Part model, mm, in its own coordinate system. Face numbers are marked on the shaded views. A direction names the side the tool comes from. Coordinates: 2 decimals unless noted, no trailing zeros. Loops run counter-clockwise (first coordinate to the right, second up) from the corner with the lowest first, then second, coordinate; pieces in that order, holes last. Notation, with made-up numbers: M 2.5,33 L 20.5,33 A17 cw 20.5,39 Z; hole C 23.25,-13.5 d2. An arc over 180 degrees is marked long. Answer as CSV lines item,"result". Start each with the question number.
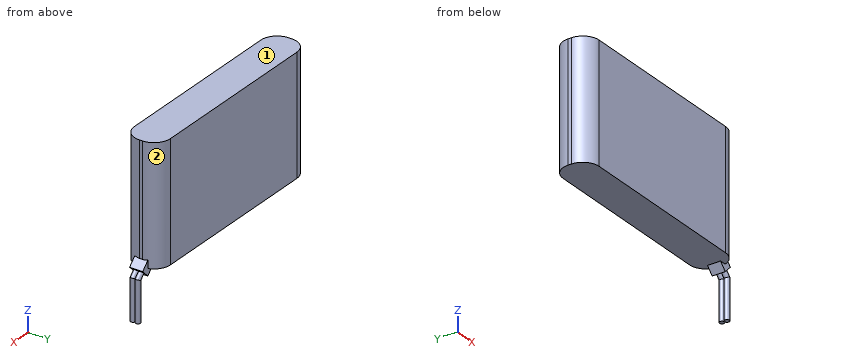
from build123d import *

# Parameters (mm, degrees)
SKETCH_1_W         = 130
SKETCH_1_H         = 72
EXTRUDE_1_DEPTH    = 22
FILLET_2_R         = 10
EXTRUDE_2_DEPTH    = 4
SWEEP_15_PROFILE_R = 1.475


with BuildPart() as part:
    # 草图1 → 凸台-拉伸1 (new body)
    with BuildSketch(Plane(origin=(0, 0, 0), x_dir=(1, 0, 0), z_dir=(0, 1, 0))):
        with Locations((2.770491803, 5.131147541)):
            Rectangle(SKETCH_1_W, SKETCH_1_H)
    extrude(amount=EXTRUDE_1_DEPTH)

    # 圆角2
    fillet_2_edges = [part.edges().sort_by_distance(p)[0] for p in [
        (67.770491803, 22, -5.131147541),
        (-62.229508197, 22, -5.131147541),
        (67.770491803, 0, -5.131147541),
        (-62.229508197, 0, -5.131147541),
    ]]
    fillet(fillet_2_edges, radius=FILLET_2_R)

    # 草图2 → 凸台-拉伸2 (add, symmetric)
    with BuildSketch(Plane(origin=(0, 11, 0), x_dir=(-1, 0, 0), z_dir=(0, -1, 0))):
        Polygon((-62.533388889, 40.348817348), (-66.98816161, 35.894044627), (-71.937909079, 40.843792095), (-67.483136357, 45.298564816), align=None)
    extrude(amount=EXTRUDE_2_DEPTH, both=True)

    # 扫描15: sweep along a path in 草图66
    with BuildLine(Plane(origin=(0, 12.5, 0), x_dir=(1, 0, 0), z_dir=(0, 1, 0))) as sweep_15_path:
        Line((69.689066092, 43.092635082), (72.470448318, 45.874017309))
        Line((72.470448318, 45.874017309), (72.470448318, 70.417467586))
    # 扫描15 profile (on start of the path) → 扫描15 (sweep)
    with BuildSketch(Plane(origin=(69.689066092, 12.5, -43.092635082), x_dir=(-0.7071067811865476, 0, -0.7071067811865476), z_dir=(0.7071067811865476, 0, -0.7071067811865476))):
        Circle(SWEEP_15_PROFILE_R)
    sweep_15 = sweep(path=sweep_15_path.line, transition=Transition.RIGHT)

    # 镜向1: 扫描15 across plane
    add(sweep_15.mirror(Plane(origin=(0, 11, 0), x_dir=(0, 0, 1), z_dir=(0, -1, 0))))


solid = part.part
Q1. Flat gauge pins, fed straight in: P1, Ø1.5, axis at y = 14.5, z = -18, coming from the -X side; P2, Ø10, axis at y = 15, z = -5, coming from the +X side; P3, Ø4, axis at y = 5, z = 20.5, coming from the -X side. Where does each tip first touch, or does it go through?
Q2. Tool access for the marked faces 1 and 2: list every direction of +Z, -Z, +X, -X, +Y, -Y with a clear straight run to the whole face (end or side of a thin tool).
Q3. Slice it at C-C, the plane y = 18.25. Write the cut outline in (x, z), and give its area (3 significant figures).
Q4. Slice it at A-A, the plane z = 7. Write the cut outline in (x, y).
Q5. Slice it at B-B, the plane x = 42. Write the cut outline in (y, z).
Q6. Wall check: L1, parallel to Z at x = -52, y = 6.5; L2, parallel to X at y = 14.75, z = 13.5; L3, parallel to Y at x = 62, z = -11.5. Give the ranges that are in metal, low to high.
Solved:
1,P1,"stops at x = -62.08"
1,P2,"stops at x = 67.77"
1,P3,"stops at x = -61.77"
2,face 1,"+Z, +X, -X, +Y, -Y"
2,face 2,"+Z, +X, +Y"
3,outline,"M -60.04,-41.13 L 65.58,-41.13 L 65.58,30.87 L -60.04,30.87 Z"
3,area,"9,040 mm2"
4,outline,"M -62.23,10 A10 ccw -52.23,0 L 57.77,0 A10 ccw 67.77,10 L 67.77,12 A10 ccw 57.77,22 L -52.23,22 A10 ccw -62.23,12 Z"
5,outline,"M 0,-41.13 L 22,-41.13 L 22,30.87 L 0,30.87 Z"
6,L1,"z = -41.13 to 30.87"
6,L2,"x = -61.84 to 67.38"
6,L3,"y = 0.94 to 21.06"
